For this review, take the finished solid that the model builds, in its own axes (mm). Face numbers are marked on the shaded views. A direction names the side the tool comes from. Give positions to 0.01 mm unless a question says otherwise; leave off trailing zeros. Order: outer loops, then holes, each group sorted by start corner. A loop starts at its lowest first (then second) coordinate and runs counter-clockwise, first axis right, second up. Notation, with made-up numbers: (85.25, -20) - (94.25, -20) arc R25 cw to (94.25, -8) - close; hole circle Ø9 at (9.5, 76.25). An arc over 180 degrees is marked (long way). Put each result on its own line as item: value. Start each with the question number.
```python
from build123d import *

# Parameters (mm, degrees)
SKICA1_W                 = 30
SKICA1_H                 = 30
P_IDAT_VYSUNUT_M1_DEPTH  = 5
SKICA2_W                 = 30
SKICA2_H                 = 30
P_IDAT_VYSUNUT_M2_DEPTH  = 5
ODEBRAT_VYSUNUT_M1_DEPTH = 30
ODEBRAT_VYSUNUT_M2_DEPTH = 30
SKICA7_W                 = 7
SKICA7_H                 = 2.5
ODEBRAT_VYSUNUT_M3_DEPTH = 30
SKICA10_R                = 8.05
SKICA10_R_2              = 6.05
P_IDAT_VYSUNUT_M7_DEPTH  = 30
SKICA13_W                = 7
SKICA13_H                = 3
ODEBRAT_VYSUNUT_M5_DEPTH = 2.5
SKICA15_R                = 2.35
ODEBRAT_VYSUNUT_M6_DEPTH = 1.7
SKICA16_W                = 3.5
SKICA16_H                = 5
P_IDAT_VYSUNUT_M8_DEPTH  = 5
ODEBRAT_VYSUNUT_M7_DEPTH = 0.8
ZAOBLIT1_R               = 4
ZAOBLIT2_R               = 4
ODEBRAT_VYSUNUT_M8_DEPTH = 5


with BuildPart() as part:
    # Skica1 → Přidat vysunutím1 (new body)
    with BuildSketch(Plane.XY):
        with Locations((-15, -15)):
            Rectangle(SKICA1_W, SKICA1_H)
    extrude(amount=P_IDAT_VYSUNUT_M1_DEPTH)

    # Skica2 → Přidat vysunutím2 (add)
    with BuildSketch(Plane(origin=(0, 0, 0), x_dir=(-1, 0, 0), z_dir=(0, 0, -1))):
        with Locations((15, -15)):
            Rectangle(SKICA2_W, SKICA2_H)
    extrude(amount=P_IDAT_VYSUNUT_M2_DEPTH)

    # Skica4 → Odebrat vysunutím1 (cut)
    with BuildSketch(Plane(origin=(0, -30, 0), x_dir=(-1, 0, 0), z_dir=(0, -1, 0))):
        with BuildLine():
            Line((30, -5), (30, 5))
            ThreePointArc((30, 5), (28.123635209, 0), (30, -5))
        make_face()
    extrude(amount=-ODEBRAT_VYSUNUT_M1_DEPTH, mode=Mode.SUBTRACT)

    # Skica5 → Odebrat vysunutím2 (cut)
    with BuildSketch(Plane(origin=(0, -30, 0), x_dir=(-1, 0, 0), z_dir=(0, -1, 0))):
        with BuildLine():
            ThreePointArc((0, -5), (1.909830056, 0), (0, 5))
            Line((0, 5), (0, -5))
        make_face()
    extrude(amount=-ODEBRAT_VYSUNUT_M2_DEPTH, mode=Mode.SUBTRACT)

    # Skica7 → Odebrat vysunutím3 (cut)
    with BuildSketch(Plane(origin=(0, 0, 0), x_dir=(1, 0, 0), z_dir=(0, 1, 0))):
        with Locations((-15, 1.25)):
            Rectangle(SKICA7_W, SKICA7_H)
    extrude(amount=-ODEBRAT_VYSUNUT_M3_DEPTH, mode=Mode.SUBTRACT)

    # Skica10 → Přidat vysunutím7 (add)
    # profile 1 of 2: a face of its own
    with BuildSketch(Plane.XZ.offset(30)):
        with Locations((-35, -1.308922253)):
            Circle(SKICA10_R)
        with Locations((-35, -1.308922253)):
            Circle(SKICA10_R_2, mode=Mode.SUBTRACT)
    # profile 2 of 2: a face of its own
    with BuildSketch(Plane.XZ.offset(30)):
        with Locations((5, -1.308922253)):
            Circle(SKICA10_R)
        with Locations((5, -1.308922253)):
            Circle(SKICA10_R_2, mode=Mode.SUBTRACT)
    extrude(amount=-P_IDAT_VYSUNUT_M7_DEPTH)

    # Skica13 → Odebrat vysunutím5 (cut)
    with BuildSketch(Plane(origin=(0, 0, -5), x_dir=(-1, 0, 0), z_dir=(0, 0, -1))):
        with Locations((15, -19)):
            Rectangle(SKICA13_W, SKICA13_H)
        with Locations((15, -11)):
            Rectangle(SKICA13_W, SKICA13_H)
    extrude(amount=-ODEBRAT_VYSUNUT_M5_DEPTH, mode=Mode.SUBTRACT)

    # Skica15 → Odebrat vysunutím6 (cut)
    with BuildSketch(Plane.XY.offset(-2.5)):
        with Locations((-15, -25.25)):
            Circle(SKICA15_R)
        with Locations(Location((-15, -4.75, 0), (0, 0, 180))):
            Circle(SKICA15_R)
    extrude(amount=-ODEBRAT_VYSUNUT_M6_DEPTH, mode=Mode.SUBTRACT)

    # Skica16 → Přidat vysunutím8 (add)
    with BuildSketch(Plane(origin=(0, 0, -5), x_dir=(-1, 0, 0), z_dir=(0, 0, -1))):
        with Locations((13.25, -15)):
            Rectangle(SKICA16_W, SKICA16_H)
        with Locations((16.75, -15)):
            Rectangle(SKICA16_W, SKICA16_H)
    extrude(amount=-P_IDAT_VYSUNUT_M8_DEPTH)

    # Skica16<3> → Odebrat vysunutím7 (cut)
    with BuildSketch(Plane(origin=(0, 0, -5), x_dir=(-1, 0, 0), z_dir=(0, 0, -1))):
        with BuildLine():
            ThreePointArc((16, -4.75), (15.707106781, -4.042893219), (15, -3.75))
            Line((15, -3.75), (15, -5.75))
            ThreePointArc((15, -5.75), (15.707106781, -5.457106781), (16, -4.75))
        make_face()
        with BuildLine():
            Line((15, -5.75), (15, -3.75))
            ThreePointArc((15, -3.75), (14, -4.75), (15, -5.75))
        make_face()
        with BuildLine():
            ThreePointArc((15, -24.25), (14, -25.25), (15, -26.25))
            Line((15, -26.25), (15, -24.25))
        make_face()
        with BuildLine():
            Line((15, -24.25), (15, -26.25))
            ThreePointArc((15, -26.25), (15.707106781, -25.957106781), (16, -25.25))
            ThreePointArc((16, -25.25), (15.707106781, -24.542893219), (15, -24.25))
        make_face()
    extrude(amount=-ODEBRAT_VYSUNUT_M7_DEPTH, mode=Mode.SUBTRACT)

    # Zaoblit1
    zaoblit1_edges = [part.edges().sort_by_distance(p)[0] for p in [
        (-15, -17.5, 0),
        (-15, -12.5, 0),
    ]]
    fillet(zaoblit1_edges, radius=ZAOBLIT1_R)

    # Zaoblit2
    # the kernel refuses this fillet: 4 mm, written as the material it takes off along each edge
    with BuildSketch(Plane(origin=(-18.5, -20.5, -2.5), x_dir=(0, 0, -1), z_dir=(1, 0, 0)), Plane(origin=(-11.5, -9.5, -2.5), x_dir=(0, 0, -1), z_dir=(-1, 0, 0))) as zaoblit2_piece_1:
        with BuildLine():
            CenterArc((4, -3.708099244), ZAOBLIT2_R, 112.024312837, 67.975687163)
            Line((0, -3.708099244), (-0.08, -3.708099244))
            Line((-0.08, -3.708099244), (-0.08, 0))
            Line((-0.08, 0), (0, 0.08))
            ThreePointArc((0, 0.08), (1.25, 0.08), (2.47, 0.074161985))
            Line((2.47, 0.074161985), (2.5, 0))
        make_face()
    extrude(amount=7, mode=Mode.SUBTRACT)

    # Skica17 → Odebrat vysunutím8 (cut)
    with BuildSketch(Plane.XY.offset(5)):
        Polygon((-8.937822174, -15), (-11.968911087, -9.75), (-18.031088913, -9.75), (-21.062177826, -15), (-18.031088913, -20.25), (-11.968911087, -20.25), align=None)
    extrude(amount=-ODEBRAT_VYSUNUT_M8_DEPTH, mode=Mode.SUBTRACT)


solid = part.part
```
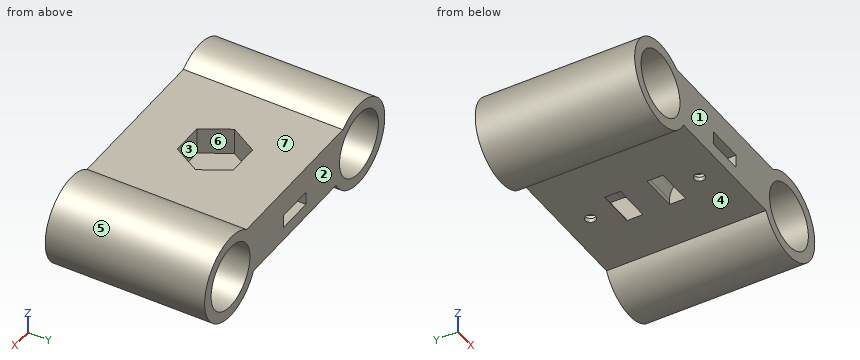
1. Add section D-D, the plane z = -8. Give the boundary of the cut face in (x, y).
2. Clearance check with flat-ended pins moving along their axes: pin 1 (4 mm diameter, centred on x = -30.5, y = -8, fed in from -Z); pin 2 (8.5 mm diameter, centred on x = -17.5, y = -15.5, fed in from +Z); pin 3 (2 mm diameter, centred on x = -14, y = -25, fed in from -Z). State where each tip first meets the part, or that it passes through.
3. Wall thickness on line 1 (X direction, y = -18, z = -1.5); line 2 (X direction, y = -4.75, z = -3); line 3 (Z direction, x = 5, y = -16.5): over which ranges is each line inside the solid? List them lowest first. Write a range as from..to.
4. Add section C-C, the plane y = -13.75. Give the boundary of the cut face in (x, z).
5. The part is to be moulded in two halves that separate along Y. For the marked faces 1, 2, 3 and 4, say which applies: released by +Y, released by -Y, zero draft, split by the parting line, or undercut.
6. Add section B-B, the plane x = -35. Give the boundary of the cut face in (y, z).
7. Tool access review of the marked faces 5, 6 and 7: name each direction out of +Z, -Z, +X, -X, +Y, -Y from which nothing blocks a thin tool from reaching the whole face with its end or side.
8. Add section A-A, the plane z = 1.5. Give the boundary of the cut face in (x, y), then the cut area to 3 significant figures.
Found:
1. outline: (-39.48, -30) - (-30.52, -30) - (-30.52, 0) - (-39.48, 0) - close; (0.52, -30) - (9.48, -30) - (9.48, 0) - (0.52, 0) - close
2. pin 1: stops at z = -8.96
2. pin 2: stops at z = 5
2. pin 3: stops at z = -5
3. line 1: x = -43.05..-41.05, -28.95..-1.05, 11.05..13.05
3. line 2: x = -42.87..-40.81, -29.19..-17.35, -12.65..-0.81, 10.81..12.87
3. line 3: z = -9.36..-7.36, 4.74..6.74
4. outline: (-30, 5) arc R8.05 ccw (long way) to (-27.85, -5) - (-2.15, -5) arc R8.05 ccw (long way) to (0, 5) - (-9.66, 5) - (-9.66, 0) - (-20.34, 0) - (-20.34, 5) - close; hole circle Ø12.1 at (-35, -1.31); hole circle Ø12.1 at (5, -1.31)
5. face 1: released by -Y
5. face 2: released by +Y
5. face 3: undercut
5. face 4: zero draft
6. outline: (-30, -9.36) - (0, -9.36) - (0, -7.36) - (-30, -7.36) - close; (-30, 4.74) - (0, 4.74) - (0, 6.74) - (-30, 6.74) - close
7. face 5: +Y, -Y
7. face 6: +Z
7. face 7: +Z, +Y, -Y
8. outline: (-42.54, -30) - (-40.36, -30) - (-40.36, 0) - (-42.54, 0) - close; (-29.64, -30) - (-0.36, -30) - (-0.36, 0) - (-29.64, 0) - close; (10.36, -30) - (12.54, -30) - (12.54, 0) - (10.36, 0) - close; hole (-21.06, -15) - (-18.03, -20.25) - (-11.97, -20.25) - (-8.94, -15) - (-11.97, -9.75) - (-18.03, -9.75) - close
8. area: 914 mm^2
